Part print with two shaded views. Sizes in mm from the minimum x, y, z corner. Coordinates: 2 decimals unless noted, no trailing zeros. Loops run counter-clockwise (first coordinate to the right, second up) from the corner with the lowest first, then second, coordinate; pieces in that order, holes last. Notation, with made-up numbers: (-4.75, 5) - (33.25, 5) arc R9 cw to (33.25, 16) - close; hole circle Ø6 at (75, -31). An arc over 180 degrees is marked (long way). Answer as CSV lines item,"result".
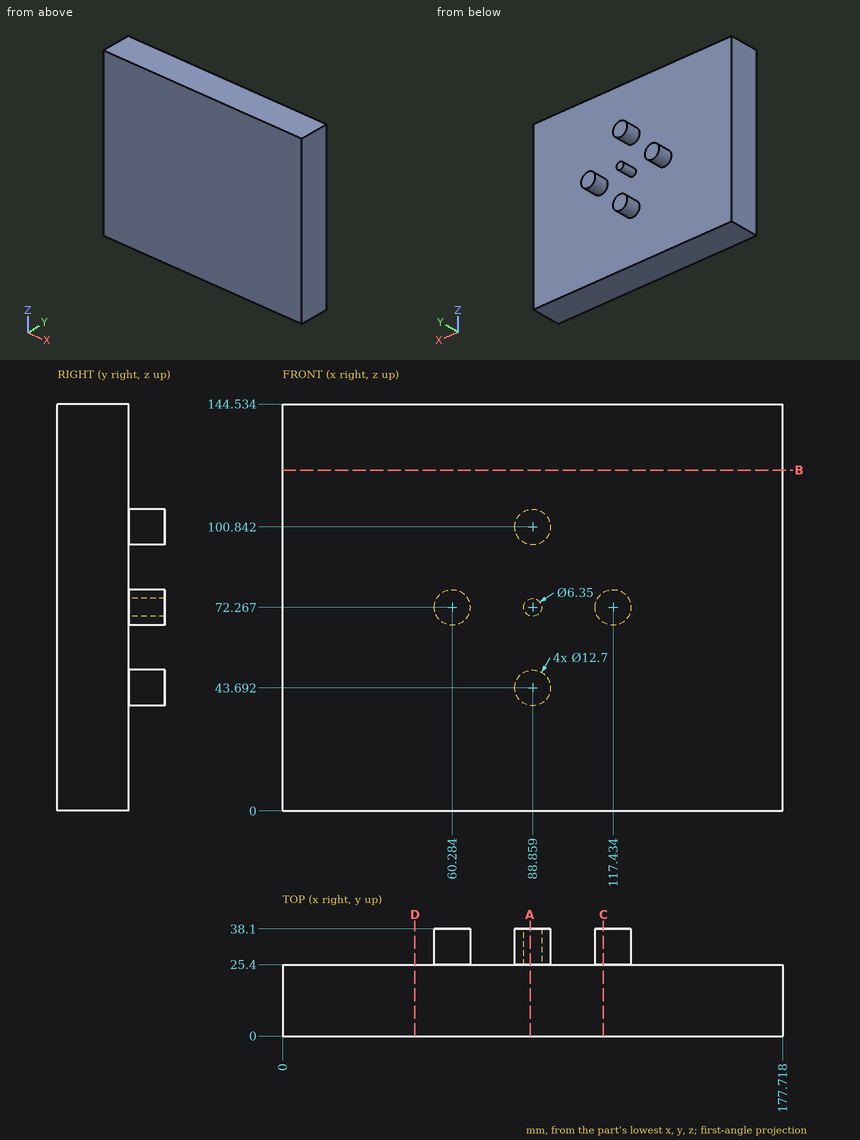
Q1. Saw through at D-D (x = 47). Give the cut face in (y, z), then the cut area to 3 significant figures.
Results:
outline,"(0, 0) - (25.4, 0) - (25.4, 144.53) - (0, 144.53) - close"
area,"3,670 mm^2"
Q2. Flat gauge pin, fed straight in: pin 1 (2 mm diameter, centred on x = 152, z = 93, fed in from +Y). Where does the tip first touch, or does it go through?
Results:
pin 1,"stops at y = 25.4"
Q3. Wall check: L1, parallel to Z at x = 89, y = 29 (1 decimal); L2, parallel to Y at x = 130, z = 37.5; L3, parallel to X at y = 27, z = 69. Give the ranges that are in metal, low to high.
Results:
L1,"z = 37.3 to 50, 69.1 to 75.4, 94.5 to 107.2"
L2,"y = 0 to 25.4"
L3,"x = 54.84 to 65.73, 111.99 to 122.88"
Q4. Saw through at B-B (z = 121). Give the cut face in (x, y), then the cut area to 3 significant figures.
Results:
outline,"(0, 0) - (177.72, 0) - (177.72, 25.4) - (0, 25.4) - close"
area,"4,510 mm^2"
Q5. Saw through at A-A (x = 88). Give the cut face in (y, z), then the cut area to 3 significant figures.
Results:
outline,"(0, 0) - (25.4, 0) - (25.4, 37.4) - (38.1, 37.4) - (38.1, 49.98) - (25.4, 49.98) - (25.4, 69.21) - (38.1, 69.21) - (38.1, 75.32) - (25.4, 75.32) - (25.4, 94.55) - (38.1, 94.55) - (38.1, 107.13) - (25.4, 107.13) - (25.4, 144.53) - (0, 144.53) - close"
area,"4,070 mm^2"
Q6. Saw through at C-C (x = 114). Give the cut face in (y, z), then the cut area to 3 significant figures.
Results:
outline,"(0, 0) - (25.4, 0) - (25.4, 66.93) - (38.1, 66.93) - (38.1, 77.61) - (25.4, 77.61) - (25.4, 144.53) - (0, 144.53) - close"
area,"3,810 mm^2"
